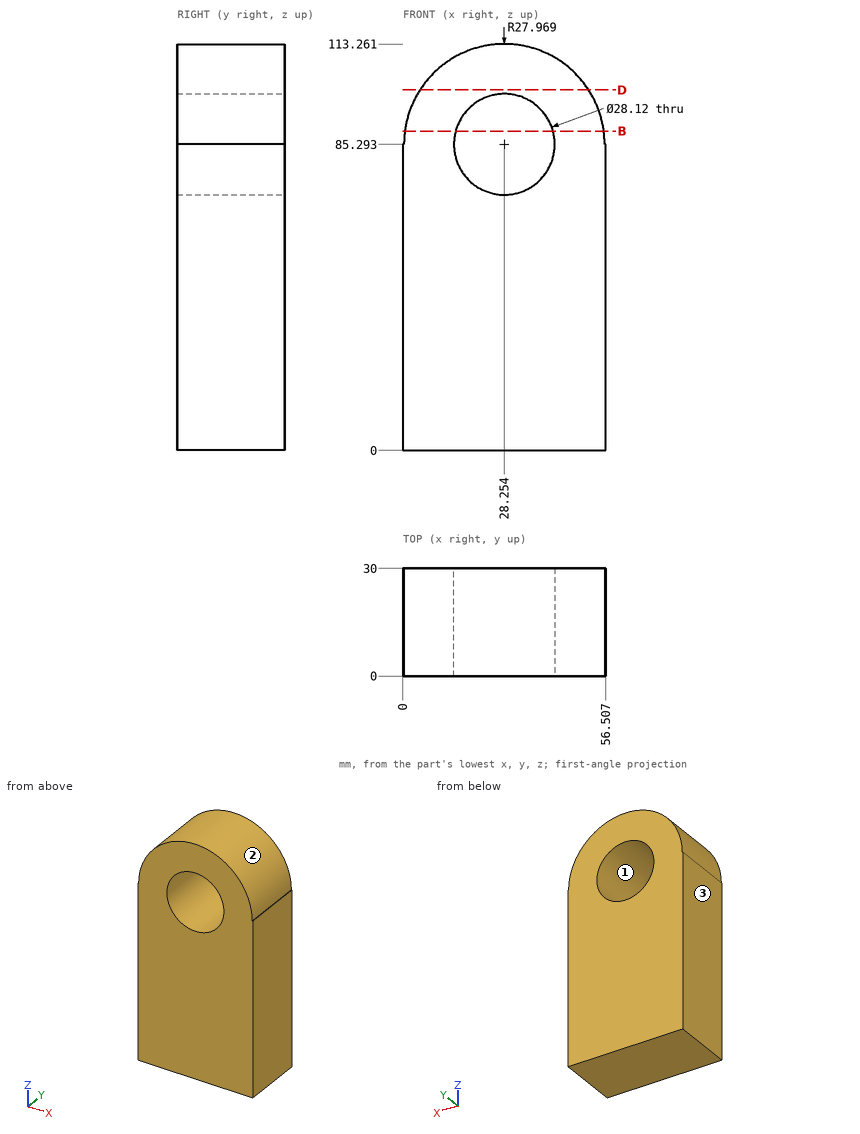
The drawing under review shows one solid part. Ordinate dimensions are in mm from its lowest x, y, z. Give positions to 0.01 mm unless a question says otherwise; leave off trailing zeros. Order: outer loops, then holes, each group sorted by start corner. A loop starts at its lowest first (then second) coordinate and runs counter-clockwise, first axis right, second up. Notation, with made-up numbers: (-5.75, -25) - (17.25, -25) arc R15 cw to (17.25, -20) - close; hole circle Ø10 at (35.25, 75.5). An arc over 180 degrees is marked (long way). Answer as a JSON object with one key per item and string values. Group by question number.
Item 1: Draft analysis for pull direction Z (two halves, no side actions). For the marked faces 1, 2 and 3, state which applies: pulls with the +Z half, pulls with the -Z half, needs draft (parallel to the pull), parting line crosses it, or undercut.
Item 2: Wall thickness on line 1 along Z through (x, y) = (30.5, 12.25); line 2 along Z through (x, y) = (17, 16.75) (1 decimal); line 3 along X through (y, z) = (8.5, 91) (1 decimal): over which ranges is each line inside the solid? List them lowest first.
Item 3: Clearance check with flat-ended pins moving along their axes: pin 1 Ø6 at (x, y) = (23, 20) entering from +Z; pin 2 Ø2 at (y, z) = (10, 80) entering from -X. State where each tip first meets the part, or that it passes through.
Item 4: Take a section at B-B on z = 89. Give the boundary of the cut face in (x, y) (1 decimal).
Item 5: Take a section at D-D on z = 100.5. Give the boundary of the cut face in (x, y), and give its area (3 significant figures).
Reported:
{
 "1": {"face 1": "undercut", "face 2": "pulls with the +Z half", "face 3": "needs draft"},
 "2": {"line 1": "0 to 71.41, 99.17 to 113.17", "line 2": "0 to 76.9, 93.7 to 110.9", "line 3": "0.9 to 15.4, 41.1 to 55.6"},
 "3": {"pin 1": "z = 113.17", "pin 2": "x = 0"},
 "4": {"outline": "(0.5, 0) - (14.7, 0) - (14.7, 30) - (0.5, 30) - close; (41.8, 0) - (56, 0) - (56, 30) - (41.8, 30) - close"},
 "5": {"outline": "(4.78, 0) - (51.73, 0) - (51.73, 30) - (4.78, 30) - close", "area": "1,410 mm^2"}
}
